```python
from build123d import *

# Parameters (mm, degrees)
F1_DEPTH = 60
F3_DEPTH = 60.001
F5_DEPTH = 100.001


with BuildPart() as f1:
    # F0 (on Top) → F1 (new body)
    with BuildSketch(Plane.XY):
        Polygon((0, 60), (0, 0), (20, 0), (20, 15), (55, 15), (55, 0), (70, 0), (70, 20), (100, 20), (100, 60), align=None)
    extrude(amount=F1_DEPTH)

    # F2 (on Front) → F3 (cut, through all)
    with BuildSketch(Plane.XZ):
        Polygon((100, 60), (75.033442, 60), (100, 35.033442), align=None)
        Polygon((15.358984, 40), (50, 60), (0, 60), (0, 40), align=None)
    extrude(amount=-F3_DEPTH, mode=Mode.SUBTRACT)

    # F4 (on Right) → F5 (cut, through all)
    with BuildSketch(Plane.YZ):
        Polygon((20, 27), (50, 60), (20, 60), align=None)
        Polygon((20, 27), (20, 60), (0, 60), (0, 5), align=None)
    extrude(amount=F5_DEPTH, mode=Mode.SUBTRACT)


solid = f1.part
```
Input: part model. Units: mm. Frame: model coordinates. A direction names the side the tool comes from. Give positions to 0.01 mm unless a question says otherwise; leave off trailing zeros. Write each loop counter-clockwise with the first axis right and the second up, starting at its lowest first coordinate (ties: lowest second). Pieces come first, ordered by that corner, then holes. Notation, with made-up numbers: (88, -40) - (130, -40) arc R14 cw to (130, -23) - close; hole circle Ø7 at (3, -35.75). An arc over 180 degrees is marked (long way). Write item = value, one per line. Start each with the question number.
1. Section query D-D, the plane x = 90. Output: boundary loops of the cut face in (y, z).
2. Access query for faces 1 (the flat face through (8, 46, 40)), 2 (the flat face through (55, 9, 8)), 3 (the flat face through (62, 55, 60)). Directions: +Z, -Z, +X, -X, +Y, -Y. A direction counts if a zero-diameter tool reaches every point of the face in a straight line with its end or side. Return the directions, or none.
3. Section query A-A, the plane y = 7. Output: boundary loops of the cut face in (x, z).
4. Section query B-B, the plane y = 51.5. Output: boundary loops of the cut face in (x, z).
5. Section query C-C, the plane z = 15. Output: boundary loops of the cut face in (x, y).
6. Mould query, pull axis X, two halves, no side actions, for faces 4 (the flat face through (85, 20, 13)), 5 (the flat face through (70, 12, 10)), 6 (the flat face through (20, 9, 8)), 7 (the flat face through (37, 15, 11)). Classes: released by +X, released by -X, zero draft, split by the parting line, or undercut.
7. First-contact query: pin 1 Ø6.5 at (x, z) = (35, 5.5) entering from -Y; pin 2 Ø2 at (x, y) = (30.5, 40) entering from +Z; pin 3 Ø7.5 at (x, y) = (11, 46) entering from +Z. Flat tips, straight axial feed; report the tip coordinate or a pass-through.
8. Ray query, L1, parallel to X at y = 7, z = 6; L2, parallel to Y at x = 39.5, z = 6.5; L3, parallel to Y at x = 78, z = 21.5. Return the intervals inside material, ascending.
Check sheet entries:
q1.outline = (20, 0) - (60, 0) - (60, 45.03) - (36.39, 45.03) - (20, 27) - close
q2.face_1 = +Z, -X, +Y, -Y
q2.face_2 = +Z, -Z, -Y
q2.face_3 = +Z, +X, -X, +Y, -Y
q3.outline = (0, 0) - (20, 0) - (20, 12.7) - (0, 12.7) - close; (55, 0) - (70, 0) - (70, 12.7) - (55, 12.7) - close
q4.outline = (0, 0) - (100, 0) - (100, 35.03) - (75.03, 60) - (50, 60) - (15.36, 40) - (0, 40) - close
q5.outline = (0, 9.09) - (20, 9.09) - (20, 15) - (55, 15) - (55, 9.09) - (70, 9.09) - (70, 20) - (100, 20) - (100, 60) - (0, 60) - close
q6.face_4 = zero draft
q6.face_5 = released by +X
q6.face_6 = undercut
q6.face_7 = undercut
q7.pin_1 = 15
q7.pin_2 = 49.3
q7.pin_3 = 40
q8.L1 = 0 to 20, 55 to 70
q8.L2 = 15 to 60
q8.L3 = 20 to 60
